Job drawing, mm, ordinate dimensions from the low corner. One solid piece. A direction names the side the tool comes from. Round coordinates to 2 decimals unless told otherwise and drop trailing zeros. Loops run counter-clockwise (first coordinate to the right, second up) from the corner with the lowest first, then second, coordinate; pieces in that order, holes last.
1) Drop flat-ended pins along their axis: P1, Ø2, axis at x = 39.5, y = 27, coming from the +Z side; P2, Ø1.5, axis at y = 28.5, z = 3, coming from the -X side; P3, Ø3, axis at x = 27, z = 9, coming from the -Y side; P4, Ø1.5, axis at x = 32.5, y = 31.5, coming from the +Z side. Give the stop position or say it passes through.
2) Band-saw the part on D-D, the plane z = 13.25. Write the cut outline in (x, y).
3) 3-axis set-ups, long thin cutter, end or side, ignore diameter. For the marked faces 1 and 2: which of +Z, -Z, +X, -X, +Y, -Y reach the whole face in a straight line?
4) Band-saw the part on B-B, the plane x = 22.86. Write the cut outline in (y, z) (3 decimals).
5) Band-saw the part on A-A, the plane z = 9. Write the cut outline in (x, y) (3 decimals), then the cut area to 3 significant figures.
6) Probe line 1 (Y direction, x = 22.86, z = 7) (3 decimals); line 2 (X direction, y = 12, z = 3.5); line 3 (Y direction, x = 32, z = 11.5). List the from-to ranges inside material, lowest first.
7) Mould opens along Y. For the marked faces 3, 4 and 5 say: +Y half, -Y half, draft (parallel to the pull), parting line (faces both ways), or undercut.
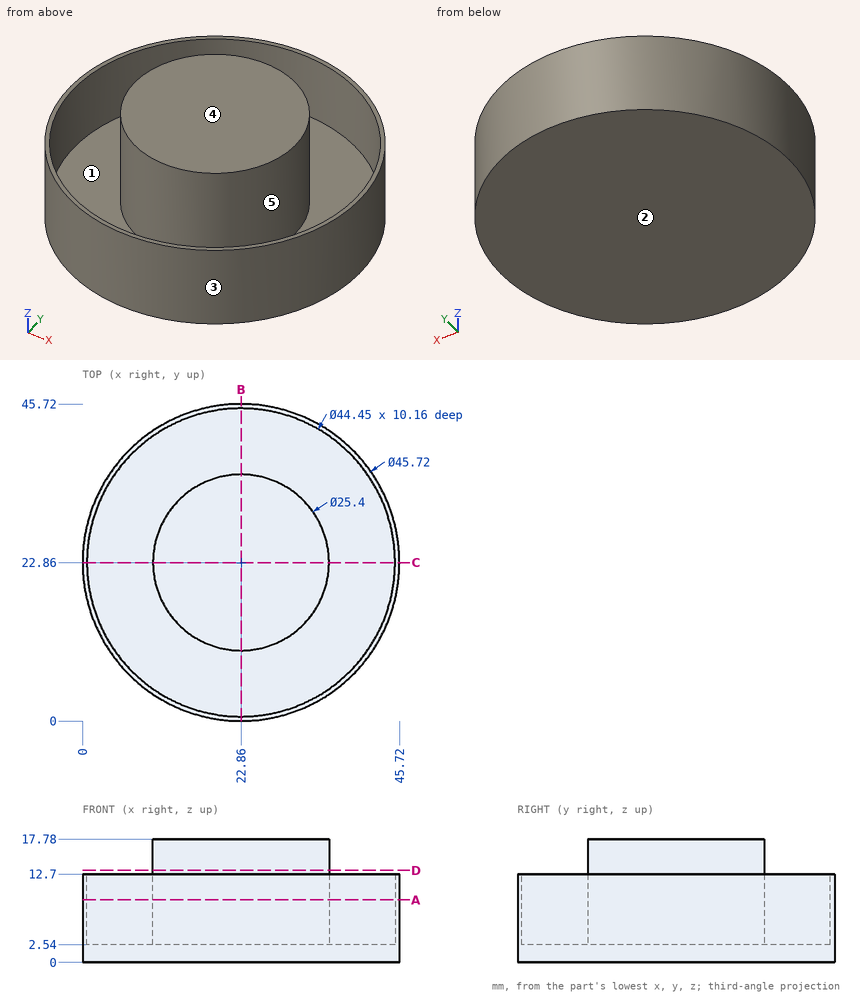
Reported:
1. P1: stops at z = 2.54
1. P2: stops at x = 0.53
1. P3: stops at y = 0.15
1. P4: stops at z = 17.78
2. outline: circle Ø25.4 at (22.86, 22.86)
3. face 1: +Z
3. face 2: -Z, +X, -X, +Y, -Y
4. outline: (0, 0) - (45.72, 0) - (45.72, 12.7) - (45.085, 12.7) - (45.085, 2.54) - (35.56, 2.54) - (35.56, 17.78) - (10.16, 17.78) - (10.16, 2.54) - (0.635, 2.54) - (0.635, 12.7) - (0, 12.7) - close
5. outline: circle Ø45.72 at (22.86, 22.86); circle Ø25.4 at (22.86, 22.86); hole circle Ø44.45 at (22.86, 22.86)
5. area: 597 mm2
6. line 1: y = 0 to 0.635, 10.16 to 35.56, 45.085 to 45.72
6. line 2: x = 2.74 to 3.47, 16.28 to 29.44, 42.25 to 42.98
6. line 3: y = 1.91 to 2.6, 14.04 to 31.68, 43.12 to 43.81
7. face 3: parting line
7. face 4: draft
7. face 5: undercut
